Geometry check sheet. Reference: the model listing, model coordinates, mm. Face numbers are marked on the shaded views. A direction names the side the tool comes from. Round coordinates to 2 decimals unless told otherwise and drop trailing zeros. Loops run counter-clockwise (first coordinate to the right, second up) from the corner with the lowest first, then second, coordinate; pieces in that order, holes last.
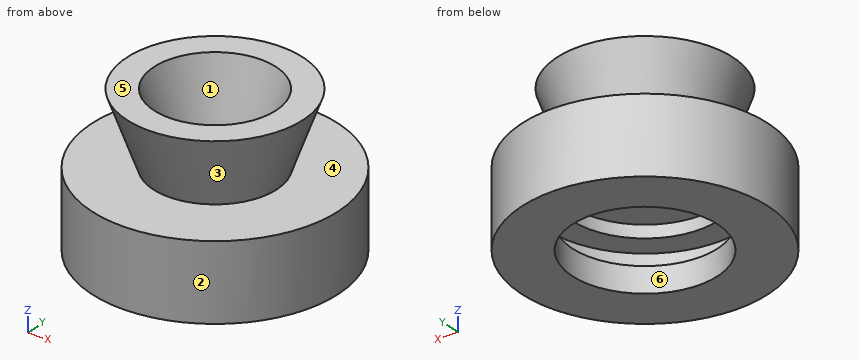
```python
from build123d import *

# Parameters (mm, degrees)
ESBO_O1_R                = 9.75
RESSALTO_EXTRUS_O1_DEPTH = 6
CASCA9_T                 = -2
ESBO_O3_R                = 2.045070657
CORTE_EXTRUS_O2_DEPTH    = 17.860255581
ESBO_O4_R                = 5.75
CORTE_EXTRUS_O3_DEPTH    = 5


with BuildPart() as part:
    # Esboço1 → Ressalto-extrusão1 (new body)
    with BuildSketch(Plane.XY):
        Circle(ESBO_O1_R)
    extrude(amount=-RESSALTO_EXTRUS_O1_DEPTH)

    # Esboço2 → Revolução1 (revolve)
    with BuildSketch(Plane(origin=(0, 0, 0), x_dir=(1, 0, 0), z_dir=(0, 1, 0)), mode=Mode.PRIVATE) as revolu_o1_sk:
        Polygon((0, 0), (-4.896169564, 0), (-6.960749361, -5.702742821), (0, -5.702742821), align=None)
    revolve(revolu_o1_sk.sketch.rotate(Axis((0, 0, 5.702742821), (0, 0, -1)), 180), axis=Axis((0, 0, 5.702742821), (0, 0, -1)))

    # Casca9
    casca9_openings = [part.faces().sort_by_distance(p)[0] for p in [
        (0, 0, 5.702742821),
    ]]
    offset(amount=CASCA9_T, openings=casca9_openings, kind=Kind.INTERSECTION)

    # Esboço3 → Corte-extrusão2 (cut, through all)
    with BuildSketch(Plane.XY.offset(-4)):
        Circle(ESBO_O3_R)
    extrude(amount=-CORTE_EXTRUS_O2_DEPTH, mode=Mode.SUBTRACT)

    # Esboço4 → Corte-extrusão3 (cut)
    with BuildSketch(Plane(origin=(0, 0, -6), x_dir=(-1, 0, 0), z_dir=(0, 0, -1))):
        Circle(ESBO_O4_R)
    extrude(amount=-CORTE_EXTRUS_O3_DEPTH, mode=Mode.SUBTRACT)


solid = part.part
```
1) Mould release check, pull along Z, two halves, no side actions. Record for the marked faces 1, 2 and 3: +Z half, -Z half, draft (parallel to the pull), parting line (faces both ways), or undercut.
Report:
face 1: +Z half
face 2: draft
face 3: undercut
2) Scan lines: line 1 along Y through (x, z) = (0, -3.45); line 2 along Y through (x, z) = (0, -4.8); line 3 along Z through (x, y) = (-4.75, -5.5). Record each from-to range of solid material in increasing order.
Report:
line 1: y = -9.75 to -7.75, 7.75 to 9.75
line 2: y = -9.75 to -5.75, 5.75 to 9.75
line 3: z = -6 to -4, -2 to 0
3) Sectioned sample at C-C, the plane x = 6.5. State how many separate pieces and enclosed holes the cut face has, then the cut area to 3 significant figures.
Report:
separate pieces: 2
enclosed holes: 1
area: 74.5 mm2
4) Sectioned sample at A-A, the plane x = 0. Record the cut outline in (y, z), then the cut area to 3 significant figures.
Report:
outline: (-9.75, -6) - (-5.75, -6) - (-5.75, -4) - (-7.75, -4) - (-7.75, -2) - (-5.75, -2) - (-5.75, -1) - (-2.41, -1) - (-4.83, 5.7) - (-6.96, 5.7) - (-4.9, 0) - (-9.75, 0) - close; (2.41, -1) - (5.75, -1) - (5.75, -2) - (7.75, -2) - (7.75, -4) - (5.75, -4) - (5.75, -6) - (9.75, -6) - (9.75, 0) - (4.9, 0) - (6.96, 5.7) - (4.83, 5.7) - close
area: 70.6 mm2
5) Gauge pin test, flat ends, axial feed: pin 1 (3 mm diameter, centred on x = 2.5, y = 1.5, fed in from -Z); pin 2 (1.5 mm diameter, centred on y = -7, z = -4.5, fed in from +X); pin 3 (1 mm diameter, centred on x = -5, z = 0, fed in from +Y). Record the tip position at first contact, or that the pin passes through.
Report:
pin 1: stops at z = -1
pin 2: stops at x = 7.48
pin 3: stops at y = 8.65
6) Access from +Z, -Z, +X, -X, +Y, -Y to the whole of each face (thin tool, end or side, straight path). Record for the marked faces 4, 5 and 6.
Report:
face 4: none
face 5: +Z, +X, -X, +Y, -Y
face 6: -Z
7) Sectioned sample at D-D, the plane z = -3.5. Record the cut outline in (x, y).
Report:
outline: circle Ø19.5 at (0, 0); hole circle Ø15.5 at (0, 0)
